from build123d import *

# Parameters (mm, degrees)
BOSS_EXTRUDE1_DEPTH = 1
SKETCH2_W           = 66.2
SKETCH2_H           = 25
BOSS_EXTRUDE2_DEPTH = 3
SKETCH3_W           = 0.3
SKETCH3_H           = 15
SKETCH3_W_2         = 40
SKETCH3_H_2         = 0.3
BOSS_EXTRUDE3_DEPTH = 1.6
FILLET1_START       = 1
FILLET1_DEPTH       = 70.2
FILLET1_2_DEPTH     = 31


with BuildPart() as part:
    # Sketch1 → Boss-Extrude1 (new body)
    with BuildSketch(Plane.XY):
        with BuildLine():
            Line((1, 0), (71.2, 0))
            ThreePointArc((71.2, 0), (71.907106781, 0.292893219), (72.2, 1))
            Line((72.2, 1), (72.2, 30))
            ThreePointArc((72.2, 30), (71.907106781, 30.707106781), (71.2, 31))
            Line((71.2, 31), (1, 31))
            ThreePointArc((1, 31), (0.292893219, 30.707106781), (0, 30))
            Line((0, 30), (0, 1))
            ThreePointArc((0, 1), (0.292893219, 0.292893219), (1, 0))
        make_face()
    extrude(amount=BOSS_EXTRUDE1_DEPTH)

    # Sketch2 → Boss-Extrude2 (add)
    with BuildSketch(Plane.XY.offset(1)):
        with BuildLine():
            Line((1.5, 30), (70.7, 30))
            ThreePointArc((70.7, 30), (71.053553391, 29.853553391), (71.2, 29.5))
            Line((71.2, 29.5), (71.2, 1.5))
            ThreePointArc((71.2, 1.5), (71.053553391, 1.146446609), (70.7, 1))
            Line((70.7, 1), (1.5, 1))
            ThreePointArc((1.5, 1), (1.146446609, 1.146446609), (1, 1.5))
            Line((1, 1.5), (1, 29.5))
            ThreePointArc((1, 29.5), (1.146446609, 29.853553391), (1.5, 30))
        make_face()
        with Locations((36.1, 15.5)):
            Rectangle(SKETCH2_W, SKETCH2_H, mode=Mode.SUBTRACT)
    extrude(amount=BOSS_EXTRUDE2_DEPTH)

    # Sketch3 → Boss-Extrude3 (add)
    with BuildSketch(Plane.XY.offset(4)):
        with Locations((71.35, 15.5)):
            Rectangle(SKETCH3_W, SKETCH3_H)
        with Locations((36.1, 30.15)):
            Rectangle(SKETCH3_W_2, SKETCH3_H_2)
        with Locations((0.85, 15.5)):
            Rectangle(SKETCH3_W, SKETCH3_H)
        with Locations((36, 0.85)):
            Rectangle(SKETCH3_W_2, SKETCH3_H_2)
    extrude(amount=-BOSS_EXTRUDE3_DEPTH)

    # Fillet1: read off the stored shape, not the designer's step
    # Fillet1 outline → Fillet1 (cut)
    with BuildSketch(Plane.YZ.offset(FILLET1_START)):
        with BuildLine():
            ThreePointArc((29.8, 4), (30.153553391, 3.853553391), (30.3, 3.5))
            Line((30.3, 3.5), (30.3, 4))
            Line((30.3, 4), (29.8, 4))
        make_face()
        with BuildLine():
            Line((1.2, 4), (0.7, 4))
            Line((0.7, 4), (0.7, 3.5))
            ThreePointArc((0.7, 3.5), (0.846446609, 3.853553391), (1.2, 4))
        make_face()
    extrude(amount=FILLET1_DEPTH, mode=Mode.SUBTRACT)

    # Fillet1 2 outline → Fillet1 2 (cut)
    with BuildSketch(Plane(origin=(0, 0, 0), x_dir=(1, 0, 0), z_dir=(0, 1, 0))):
        with BuildLine():
            ThreePointArc((1.2, -4), (0.846446609, -3.853553391), (0.7, -3.5))
            Line((0.7, -3.5), (0.7, -4))
            Line((0.7, -4), (1.2, -4))
        make_face()
        with BuildLine():
            Line((71, -4), (71.5, -4))
            Line((71.5, -4), (71.5, -3.5))
            ThreePointArc((71.5, -3.5), (71.353553391, -3.853553391), (71, -4))
        make_face()
    extrude(amount=FILLET1_2_DEPTH, mode=Mode.SUBTRACT)


solid = part.part
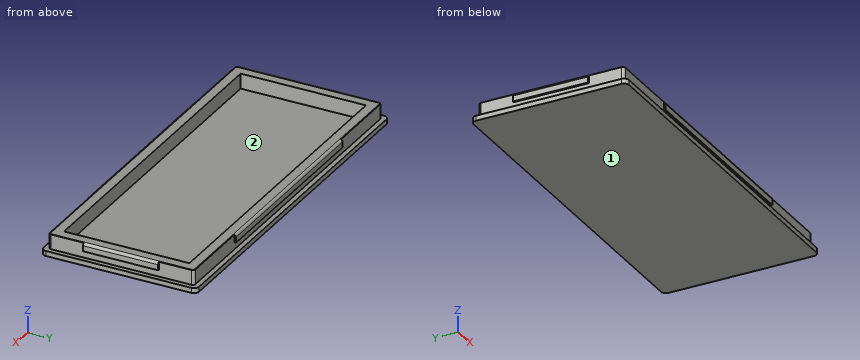
Work out the finished part from the listing and answer in its coordinate system (mm). Face numbers are marked on the shaded views. Round coordinates to 2 decimals unless told otherwise and drop trailing zeros. Loops run counter-clockwise (first coordinate to the right, second up) from the corner with the lowest first, then second, coordinate; pieces in that order, holes last. Notation, with made-up numbers: M 81.5,-11.75 L 134.5,-11.75 A23 cw 134.5,-3.75 Z; hole C 36.5,-32 d9. An arc over 180 degrees is marked long. One line per question, with ' | ' between items. Start each with the question number.
(1) A cutting plane is placed at A-A on y = 11.5. Write down the section's boundary in (x, z), plus the area to 3 significant figures.
(2) Find the intervals of material crossed by line 1 (X direction, y = 6.5, z = 2.65); line 2 (Y direction, x = 13.5, z = 1.35); line 3 (Z direction, x = 30.5, y = 13), in increasing order.
(3) A cutting plane is placed at C-C on z = 1.65. Write down the section's boundary in (x, y).
(4) Flat-ended cylindrical pins translate along their axes: pin 1 Ø1.5 at (y, z) = (22, 2.5) entering from -X; pin 2 Ø1.5 at (x, y) = (12.5, 20.5) entering from -Z; pin 3 Ø6 at (x, y) = (17.5, 7.5) entering from +Z; pin 4 Ø1 at (x, z) = (16, 2.5) entering from -Y. Find the tip coordinate at first contact, or state that the pin passes through.
(5) A cutting plane is placed at D-D on y = 6. Write down the section's boundary in (x, z), plus the area to 3 significant figures.
(6) A cutting plane is placed at B-B on x = 24.5. Write down the section's boundary in (y, z).
(7) For a pull along X with two mould halves and no side action, classify the marked faces 1 and 2 as released by +X, released by -X, zero draft, split by the parting line, or undercut.
Geometry check:
1) outline: M 0,0 L 72.2,0 L 72.2,1 L 71.2,1 L 71.2,2.4 L 71.5,2.4 L 71.5,3.5 A0.5 ccw 71,4 L 69.2,4 L 69.2,1 L 3,1 L 3,4 L 1.2,4 A0.5 ccw 0.7,3.5 L 0.7,2.4 L 1,2.4 L 1,1 L 0,1 Z | area: 85.1 mm²
2) line 1: x = 1 to 3, 69.2 to 71.2 | line 2: y = 1 to 3, 28 to 30 | line 3: z = 0 to 1
3) outline: M 1,1.5 A0.5 ccw 1.5,1 L 70.7,1 A0.5 ccw 71.2,1.5 L 71.2,29.5 A0.5 ccw 70.7,30 L 1.5,30 A0.5 ccw 1,29.5 Z; hole M 3,3 L 69.2,3 L 69.2,28 L 3,28 Z
4) pin 1: stops at x = 0.7 | pin 2: stops at z = 0 | pin 3: stops at z = 1 | pin 4: stops at y = 0.7
5) outline: M 0,0 L 72.2,0 L 72.2,1 L 71.2,1 L 71.2,3.96 A0.5 ccw 71,4 L 69.2,4 L 69.2,1 L 3,1 L 3,4 L 1.2,4 A0.5 ccw 1,3.96 L 1,1 L 0,1 Z | area: 84.2 mm²
6) outline: M 0,0 L 31,0 L 31,1 L 30,1 L 30,2.4 L 30.3,2.4 L 30.3,3.5 A0.5 ccw 29.8,4 L 28,4 L 28,1 L 3,1 L 3,4 L 1.2,4 A0.5 ccw 0.7,3.5 L 0.7,2.4 L 1,2.4 L 1,1 L 0,1 Z
7) face 1: zero draft | face 2: undercut
